Autodesk Inventor part; units mm, degrees
ref_plane "Work Plane1" through (0, 0, 0) normal (0, 1, 0) x (1, 0, 0)
ref_plane "YZ Plane" through (0, 0, 0) normal (1, 0, 0) x (0, 1, 0)
ref_plane "XZ Plane" through (0, 0, 0) normal (0, 1, 0) x (-1, 0, 0)
sketch "Sketch1" plane through (0, 0, 0) normal (1, 0, 0) x (0, 1, 0)
  circle A0 centre (0, 0) radius 3
  circle A1 centre (0, 0) radius 1.6
  dimension "d0" = 6
  dimension "d1" = 3.2
extrude "Body" add sketch "Sketch1" along normal blind 0.4
sketch "Sketch2" plane through (0, 0, 0) normal (-1, 0, 0) x (0, 0, 1)
  circle A0 centre (0, 0) radius 1.6
  circle A1 centre (0, 0) radius 3
  arc A2 (0.5953, 2.2216) -> (-0.5953, 2.2216) centre (0, 0) ccw
  line L0 (-0.4141, 1.5455) -> (-0.5953, 2.2216)
  line L1 (0, 0) -> (0, 2.3) construction
  line L2 (0.4141, 1.5455) -> (0.5953, 2.2216)
  line L3 (-0.4141, 1.5455) -> (0, 0) construction
  line L4 (0.4141, 1.5455) -> (0, 0) construction
  dimension "d4" = 4.6
  dimension "d5" = 15
extrude "Cut" cut sketch "Sketch2" against normal blind 0.4 contours A0 L0 A2 L2
fillet "Fillet1" radius 0.096 2 edges at (0.2, 2.2216, 0.5953) (0.2, 2.2216, -0.5953)
pattern_circular "Cuts" count 6 over 360 about axis through (-10, 0, 0) along (1, 0, 0) of "Cut", "Fillet1"
ref_plane "Work Plane1" through (0, 0, 0) normal (0, 1, 0) x (1, 0, 0)
equation "\"d0\" = SD2"
equation "\"d1\" = SD1"
equation "\"d2\" = SD"
equation "\"d4\" = 0.5 * SD2 + 0.5 * SD1"
equation "\"d6\" = SD"
equation "\"d8\" = 0.03 * SD1"
equation "\"SD1\" = 3.2"
equation "\"SD2\" = 6"
equation "\"SD\" = 0.4"
equation "\"NND\" = 3"
properties part number "IS 5371 - B3.2" material "Steel, Mild"
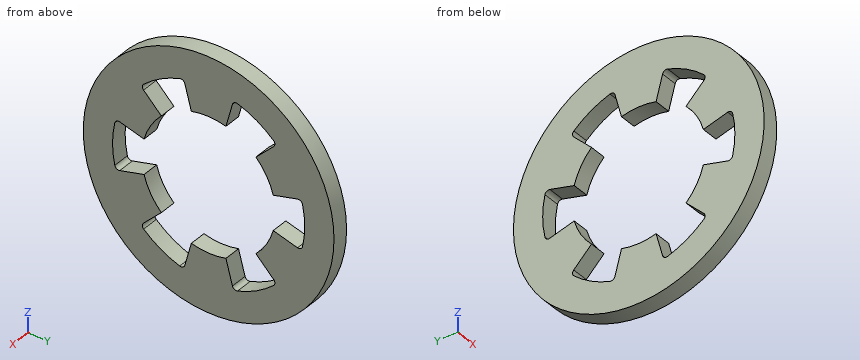
CAD build for the part. Positions are in the model's coordinates, mm. Coordinates: 2 decimals unless noted, no trailing zeros. Write each loop counter-clockwise with the first axis right and the second up, starting at its lowest first coordinate (ties: lowest second). Pieces come first, ordered by that corner, then holes.
(1) Drill centre lines: probe 1 along Y at (x, z) = (0.2, 1.8); probe 2 along Z at (x, y) = (0.05, -0.05); probe 3 along Z at (x, y) = (0.05, 1.3). Where is each one in solid material? Low to high.
(2) Cut at A-A, the plane z = 0. List the corners of the cut face in (x, y), and give its area (3 significant figures).
(3) Cut at C-C, the plane z = -1.9. List the corners of the cut face in (x, y), and give its area (3 significant figures).
(4) Cut at B-B, the plane y = 0. List the corners of the cut face in (x, z), and give its area (3 significant figures).
(5) Cut at D-D, the plane z = 2.4. List the corners of the cut face in (x, y).
Geometry says:
1. probe 1: y = -2.4 to -1.43, -0.48 to 0.48, 1.43 to 2.4
1. probe 2: z = -3 to -1.6, 1.6 to 3
1. probe 3: z = -2.7 to -1.9, -1.3 to -0.93, 0.93 to 1.3, 1.9 to 2.7
2. outline: (0, -3) - (0.4, -3) - (0.4, -2.3) - (0, -2.3) - close; (0, 2.3) - (0.4, 2.3) - (0.4, 3) - (0, 3) - close
2. area: 0.560 mm2
3. outline: (0, -2.32) - (0.4, -2.32) - (0.4, -1.3) - (0, -1.3) - close; (0, -0.51) - (0.4, -0.51) - (0.4, 0.51) - (0, 0.51) - close; (0, 1.3) - (0.4, 1.3) - (0.4, 2.32) - (0, 2.32) - close
3. area: 1.23 mm2
4. outline: (0, -3) - (0.4, -3) - (0.4, -1.6) - (0, -1.6) - close; (0, 1.6) - (0.4, 1.6) - (0.4, 3) - (0, 3) - close
4. area: 1.12 mm2
5. outline: (0, -1.8) - (0.4, -1.8) - (0.4, 1.8) - (0, 1.8) - close
